The drawing under review shows one solid part. Ordinate dimensions are in mm from its lowest x, y, z. A direction names the side the tool comes from. Coordinates: 2 decimals unless noted, no trailing zeros. Write each loop counter-clockwise with the first axis right and the second up, starting at its lowest first coordinate (ties: lowest second). Pieces come first, ordered by that corner, then holes. Notation, with made-up numbers: (58, 32.5) - (79, 32.5) arc R12 cw to (79, 54.5) - close; hole circle Ø7 at (-14, -11.5). An arc over 180 degrees is marked (long way). Use a Markdown table: item, result.
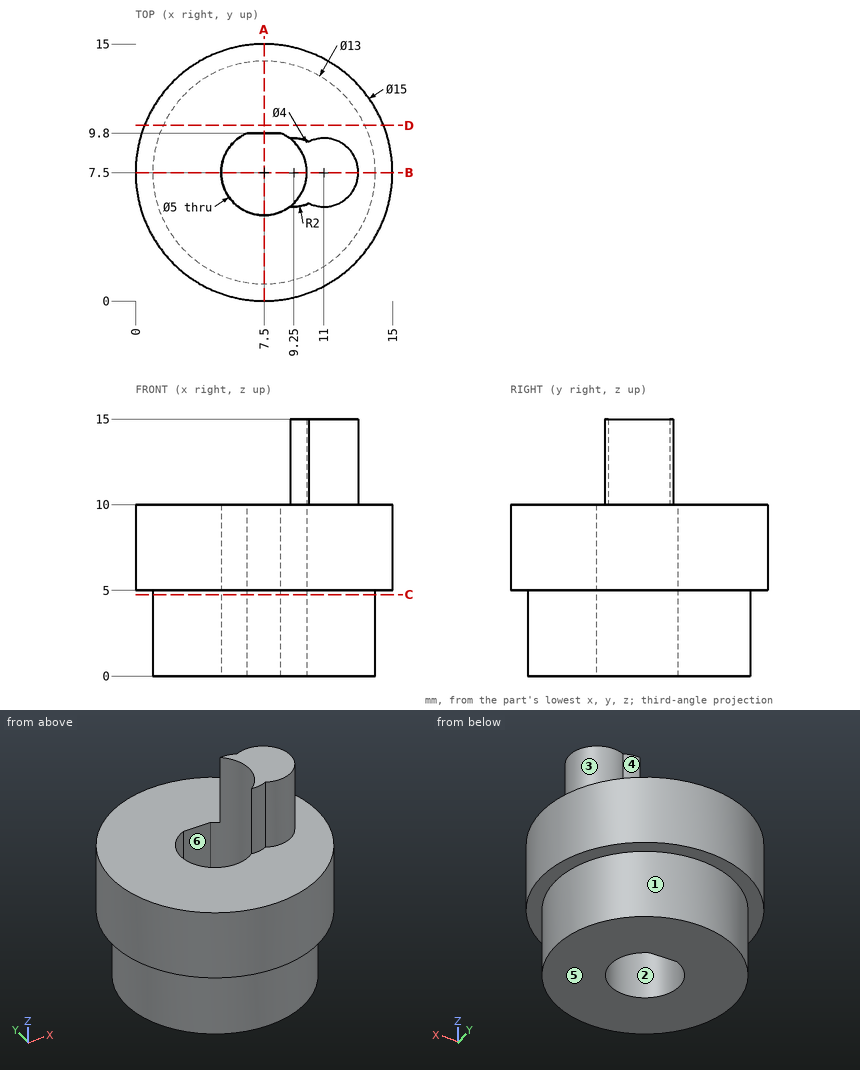
(1) Take a section at B-B on y = 7.5. Write out the cut boundary in (x, z), and give its area (3 significant figures).
Determined:
| item | result |
|---|---|
| outline | (0, 5) - (1, 5) - (1, 0) - (5, 0) - (5, 10) - (0, 10) - close; (10, 0) - (14, 0) - (14, 5) - (15, 5) - (15, 10) - (13, 10) - (13, 15) - (10, 15) - close |
| area | 105 mm2 |
(2) Draft analysis for pull direction Y (two halves, no side actions). For the marked faces 4, 5 and 6, state which applies: +Y half, -Y half, draft (parallel to the pull), parting line (faces both ways), or undercut.
Determined:
| item | result |
|---|---|
| face 4 | +Y half |
| face 5 | draft |
| face 6 | undercut |
(3) Machinability: for the marked faces 1, 2 and 3, which of the approach directions +Z, -Z, +X, -X, +Y, -Y give a long, thin tool a straight path to every point of the face, cutting with its end or side? Answer none if there is none.
Determined:
| item | result |
|---|---|
| face 1 | -Z |
| face 2 | +Z, -Z |
| face 3 | +Z |
(4) Take a section at D-D on y = 10.25. Write out the cut boundary in (x, z), and give its area (3 significant figures).
Determined:
| item | result |
|---|---|
| outline | (0.52, 5) - (1.61, 5) - (1.61, 0) - (13.39, 0) - (13.39, 5) - (14.48, 5) - (14.48, 10) - (0.52, 10) - close |
| area | 129 mm2 |
(5) Take a section at A-A on x = 7.5. Write out the cut boundary in (y, z), and give its area (3 significant figures).
Determined:
| item | result |
|---|---|
| outline | (0, 5) - (1, 5) - (1, 0) - (5, 0) - (5, 10) - (0, 10) - close; (9.8, 0) - (14, 0) - (14, 5) - (15, 5) - (15, 10) - (9.8, 10) - close |
| area | 92.0 mm2 |
(6) Take a section at C-C on z = 4.75. Write out the cut boundary in (x, y).
Determined:
| item | result |
|---|---|
| outline | circle Ø13 at (7.5, 7.5); hole (6.52, 9.8) arc R2.5 ccw (long way) to (8.48, 9.8) - close |
(7) For L1, parallel to Y at x = 7.5, z = 9.5; L2, parallel to X at y = 7.5, z = 11.75; L3, parallel to Z at x = 2.5, y = 12.75, list the stretches that pass through material, from the lowest coordinate up. Write a range as from..to.
Determined:
| item | result |
|---|---|
| L1 | 0..5, 9.8..15 |
| L2 | 10..13 |
| L3 | 5..10 |
(8) For pin 1 (5 mm diameter, centred on y = 12, z = 2, fed in from -X); pin 2 (3 mm diameter, centred on x = 6.5, z = 2, fed in from -Y); pin 3 (3 mm diameter, centred on x = 7.5, y = 7.5, fed in from -Z); pin 4 (3 mm diameter, centred on y = 3, z = 1.5, fed in from -X), all flat-tipped, find the tip position at first contact; note any pin that passes through.
Determined:
| item | result |
|---|---|
| pin 1 | x = 1.32 |
| pin 2 | y = 1 |
| pin 3 | through |
| pin 4 | x = 1.73 |
